Drawing for the job (mm, zero at the part's lowest x, y, z). Round coordinates to 2 decimals unless told otherwise and drop trailing zeros. Order: outer loops, then holes, each group sorted by start corner. A loop starts at its lowest first (then second) coordinate and runs counter-clockwise, first axis right, second up. Notation, with made-up numbers: (44.25, 56.25) - (75.25, 56.25) arc R26 ccw to (75.25, 83.25) - close; hole circle Ø10 at (-27.5, -35). An arc over 180 degrees is marked (long way). Put each result on its own line as item: value. Start each with the question number.
Item 1: Mould opens along X. For the marked faces 1 and 2 say: pulls with the +X half, pulls with the -X half, needs draft (parallel to the pull), parting line crosses it, or undercut.
Item 2: Pin check, flat tips, straight feed: pin 1 Ø2 at (y, z) = (1.5, 16) entering from +X; pin 2 Ø2 at (y, z) = (3, 28) entering from -X; pin 3 Ø1.5 at (y, z) = (2, 13) entering from -X; pin 4 Ø6 at (x, z) = (8.5, 8) entering from +Y. Stop position of each tip, or through.
Item 3: Saw through at D-D on x = 25.5. List the corners of the cut face in (y, z).
Item 4: Saw through at B-B on z = 7. List the corners of the cut face in (x, y), plus the area to 3 significant figures.
Item 5: Probe probe 1 along Z at (x, y) = (37.5, 4.75); probe 2 along X at (y, z) = (5, 48) (1 decimal); probe 3 along X at (y, z) = (2, 42.5) (1 decimal). List the from-to ranges inside material, lowest first.
Item 6: Saw through at A-A on x = 15. List the corners of the cut face in (y, z), plus the area to 3 significant figures.
Item 7: Saw through at C-C on y = 5.5. State how many separate pieces and enclosed holes the cut face has, plus the area to 3 significant figures.
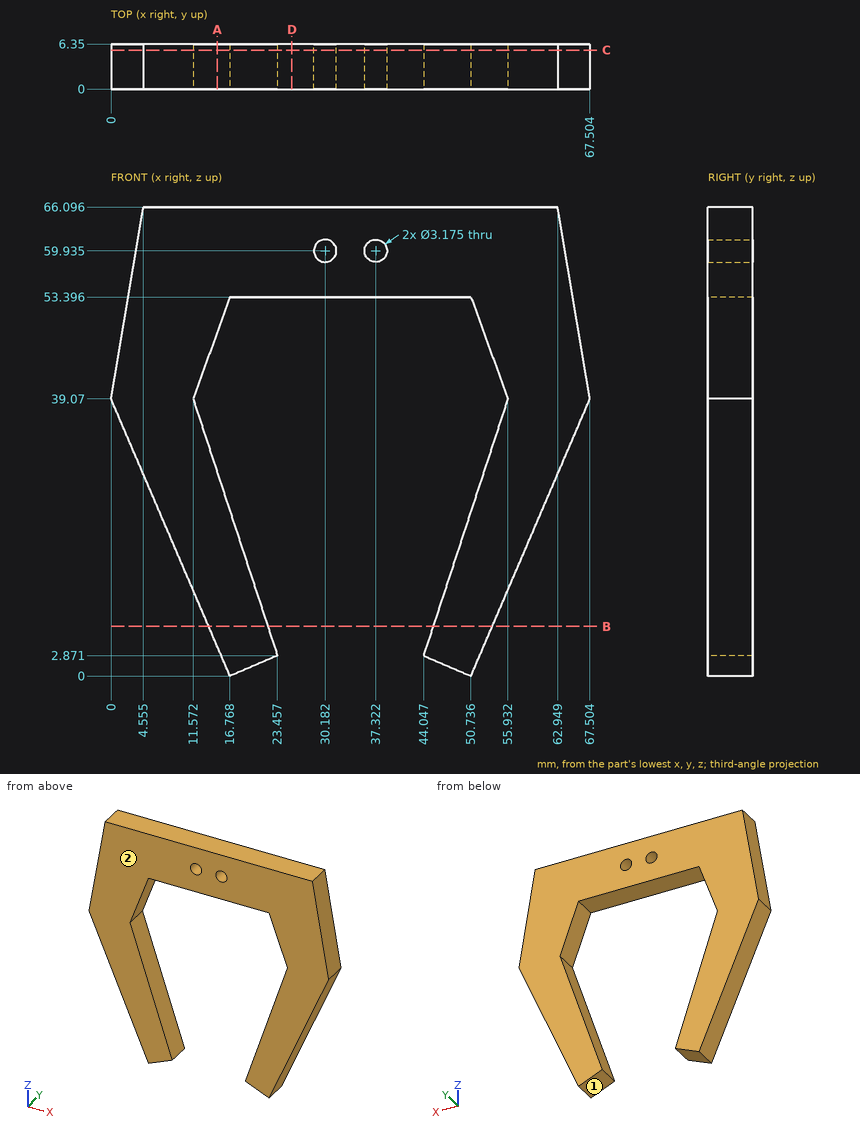
Results found:
1. face 1: undercut
1. face 2: needs draft
2. pin 1: stops at x = 58.03
2. pin 2: stops at x = 4.32
2. pin 3: stops at x = 10.87
2. pin 4: passes through
3. outline: (0, 53.4) - (6.35, 53.4) - (6.35, 66.1) - (0, 66.1) - close
4. outline: (13.76, 0) - (22.1, 0) - (22.1, 6.35) - (13.76, 6.35) - close; (45.4, 0) - (53.74, 0) - (53.74, 6.35) - (45.4, 6.35) - close
4. area: 106 mm²
5. probe 1: z = 53.4 to 58.36, 61.51 to 66.1
5. probe 2: x = 1.5 to 14.8, 52.7 to 66
5. probe 3: x = 0.6 to 12.8, 54.7 to 66.9
6. outline: (0, 4.12) - (6.35, 4.12) - (6.35, 28.63) - (0, 28.63) - close; (0, 48.52) - (6.35, 48.52) - (6.35, 66.1) - (0, 66.1) - close
6. area: 267 mm²
7. separate pieces: 1
7. enclosed holes: 2
7. area: 1,850 mm²
